Verification items for this drawing (mm, ordinates from the low corner). Coordinates: 2 decimals unless noted, no trailing zeros. Write each loop counter-clockwise with the first axis right and the second up, starting at its lowest first coordinate (ties: lowest second). Pieces come first, ordered by that corner, then holes. Notation, with made-up numbers: (89, 63) -> (96, 63) arc R26 ccw to (96, 90) -> close; hole circle Ø9 at (42, 33.5). An arc over 180 degrees is marked (long way). One line per item, written item: value. Start each with the question number.
1) Sectioned sample at C-C on x = 343. Enter the section's corners in (y, z) (1 decimal), plus the area to 3 significant figures.
2) Sectioned sample at A-A on z = 10. Enter the section's corners in (x, y), plus the area to 3 significant figures.
3) Scan lines: line 1 along Y through (x, z) = (199.5, 4) (1 decimal); line 2 along X through (y, z) = (1181, 6); line 3 along X through (y, z) = (308.5, 3). Record each from-to range of solid material in increasing order. Write a range as [from, to].
4) Sectioned sample at B-B on y = 630. Enter the section's corners in (x, z), plus the area to 3 significant figures.
5) Gauge pin test, flat ends, axial feed: P1, Ø1, axis at y = 645.5, z = 19.5, coming from the -X side; P2, Ø6, axis at x = 448, z = 33.5, coming from the +Y side; P3, Ø1.5, axis at x = 493, z = 33.5, coming from the -Y side (1 decimal). Record the tip position at first contact, or that the pin passes through.
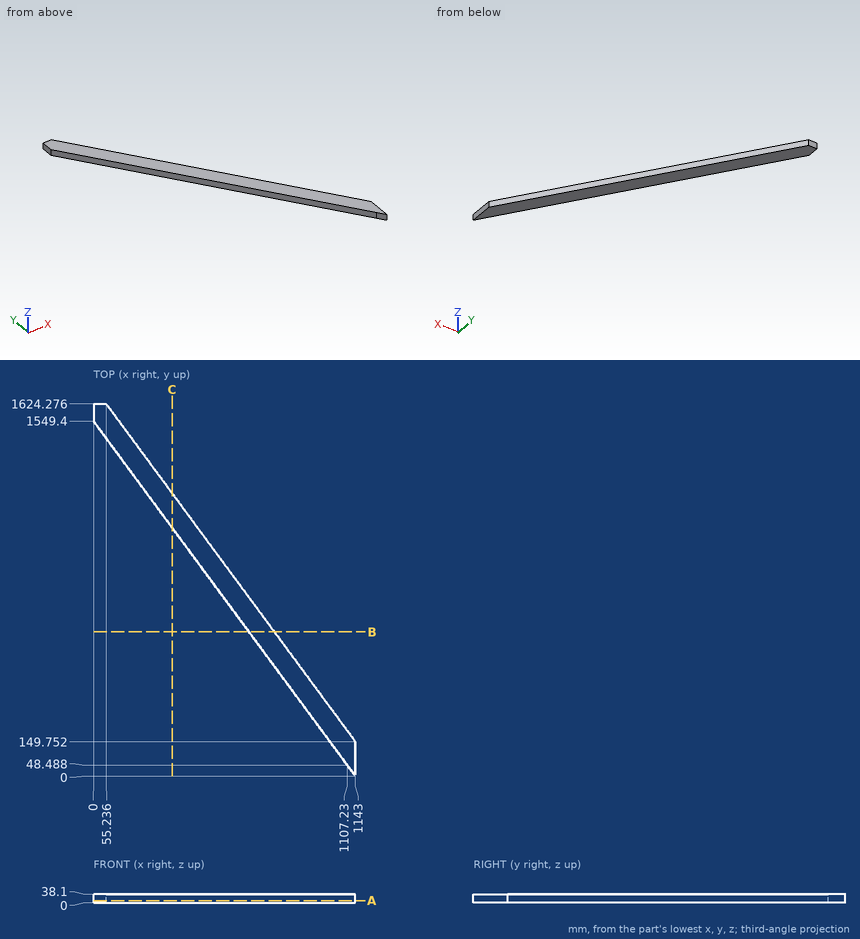
Answers:
1. outline: (1084.4, 0) -> (1234.2, 0) -> (1234.2, 38.1) -> (1084.4, 38.1) -> close
1. area: 5,710 mm2
2. outline: (0, 1549.4) -> (1107.23, 48.49) -> (1143, 0) -> (1143, 149.75) -> (55.24, 1624.28) -> (0, 1624.28) -> close
2. area: 169,000 mm2
3. line 1: y = [1279, 1428.7]
3. line 2: x = [271.77, 382.24]
3. line 3: x = [915.42, 1025.89]
4. outline: (678.25, 0) -> (788.72, 0) -> (788.72, 38.1) -> (678.25, 38.1) -> close
4. area: 4,210 mm2
5. P1: stops at x = 666.44
5. P2: stops at y = 1095.93
5. P3: stops at y = 880.1
